```python
from build123d import *

# Parameters (mm, degrees)
F1_DEPTH = 1700
F2_T     = -2.5


with BuildPart() as f1:
    # F0 (on Front) → F1 (new body)
    with BuildSketch(Plane.XZ):
        with BuildLine():
            Line((442.690637, 405), (-442.690637, 405))
            ThreePointArc((-442.690637, 405), (-600, 0), (-442.690637, -405))
            Line((-442.690637, -405), (442.690637, -405))
            ThreePointArc((442.690637, -405), (600, 0), (442.690637, 405))
        make_face()
    extrude(amount=-F1_DEPTH)

    # F2
    f2_openings = [f1.faces().sort_by_distance(p)[0] for p in [
        (0, 850, 405),
    ]]
    offset(amount=F2_T, openings=f2_openings)


solid = f1.part
```
For this review, take the finished solid that the model builds, in its own axes (mm). A direction names the side the tool comes from. Coordinates: 2 decimals unless noted, no trailing zeros. Order: outer loops, then holes, each group sorted by start corner. A loop starts at its lowest first (then second) coordinate and runs counter-clockwise, first axis right, second up. Notation, with made-up numbers: (-10.5, 81) -> (-3.5, 81) arc R13 cw to (-3.5, 98) -> close; hole circle Ø3 at (89, 49). An arc over 180 degrees is marked (long way). Answer as CSV lines item,"result".
Q1. We need section C-C (x = 164). State the section outline as (y, z) points, plus the area to 3 significant figures.
Model answer:
outline,"(0, -405) -> (1700, -405) -> (1700, 405) -> (1697.5, 405) -> (1697.5, -402.5) -> (2.5, -402.5) -> (2.5, 405) -> (0, 405) -> close"
area,"8,290 mm2"
Q2. Draft analysis for pull direction Z (two halves, no side actions). For faces 3 (the face through (-6, 838, -405)), 4 (the face through (-599.968, 838.1, 6.224)), 5 (the face through (-597.448, 838.135, 7.902)), state which applies: released by +Z, released by -Z, zero draft, split by the parting line, or undercut.
Model answer:
face 3,"released by -Z"
face 4,"split by the parting line"
face 5,"undercut"
Q3. For faces 1 (the face through (-8, 0, 6)), 2 (the face through (-8, 2.5, 7)), list the 3-axis set-ups (+Z, -Z, +X, -X, +Y, -Y) from which the entire face can be reached by the end or side of a thin tool; tool diameter is ignored.
Model answer:
face 1,"+Z, -Z, +X, -X, -Y"
face 2,"none"
Q4. Wall thickness on line 1 along Y through (x, z) = (-179, -254.5); line 2 along X through (y, z) = (961, -1); line 3 along Z through (x, y) = (202, 1513): over which ranges is each line inside the solid? List them lowest first. Write a range as [from, to].
Model answer:
line 1,"y = [0, 2.5], [1697.5, 1700]"
line 2,"x = [-600, -597.5], [597.5, 600]"
line 3,"z = [-405, -402.5]"
Q5. We need section A-A (y = 1502). State the section outline as (x, z) points.
Model answer:
outline,"(-442.69, -405) -> (442.69, -405) arc R600 ccw to (442.69, 405) -> (439.3, 405) arc R597.5 cw to (441.59, -402.5) -> (-441.59, -402.5) arc R597.5 cw to (-439.3, 405) -> (-442.69, 405) arc R600 ccw to start"
Q6. We need section D-D (z = -43). State the section outline as (x, y) points, plus the area to 3 significant figures.
Model answer:
outline,"(-598.46, 0) -> (598.46, 0) -> (598.46, 1700) -> (-598.46, 1700) -> close; hole (-595.95, 2.5) -> (595.95, 2.5) -> (595.95, 1697.5) -> (-595.95, 1697.5) -> close"
area,"14,500 mm2"
Q7. Clearance check with flat-ended pins moving along their axes: pin 1 Ø1 at (x, y) = (-97, 1118) entering from +Z; pin 2 Ø1 at (y, z) = (212.5, 33) entering from -X; pin 3 Ø2 at (y, z) = (987, -137) entering from -X; pin 4 Ø10 at (x, z) = (-53, 180.5) entering from -Y. State where each tip first meets the part, or that it passes through.
Model answer:
pin 1,"stops at z = -402.5"
pin 2,"stops at x = -599.12"
pin 3,"stops at x = -584.38"
pin 4,"stops at y = 0"
Q8. We need section B-B (z = 93). State the section outline as (x, y) points, plus the area to 3 significant figures.
Model answer:
outline,"(-592.75, 0) -> (592.75, 0) -> (592.75, 1700) -> (-592.75, 1700) -> close; hole (-590.22, 2.5) -> (590.22, 2.5) -> (590.22, 1697.5) -> (-590.22, 1697.5) -> close"
area,"14,500 mm2"
